For this review, take the finished solid that the model builds, in its own axes (mm). Face numbers are marked on the shaded views. A direction names the side the tool comes from. Give positions to 0.01 mm unless a question says otherwise; leave off trailing zeros. Write each loop counter-clockwise with the first axis right and the second up, starting at its lowest first coordinate (ties: lowest second). Pieces come first, ordered by that corner, then holes.
from build123d import *

# Parameters (mm, degrees)
SKETCH1_R           = 14
SKETCH1_R_2         = 7.5
BOSS_EXTRUDE1_DEPTH = 5
SKETCH2_R           = 13
SKETCH2_R_2         = 9
CUT_EXTRUDE1_DEPTH  = 0.05
FILLET1_R           = 0.45


with BuildPart() as part:
    # Sketch1 → Boss-Extrude1 (new, symmetric)
    with BuildSketch(Plane(origin=(0, 0, 0), x_dir=(1, 0, 0), z_dir=(0, 1, 0))):
        with Locations(Location((0, 0, 0), (0, 0, 270))):
            Circle(SKETCH1_R)
        with Locations(Location((0, 0, 0), (0, 0, 270))):
            Circle(SKETCH1_R_2, mode=Mode.SUBTRACT)
    extrude(amount=BOSS_EXTRUDE1_DEPTH, both=True)

    # Sketch2 → Cut-Extrude1 (cut)
    with BuildSketch(Plane(origin=(0, 5, 0), x_dir=(1, 0, 0), z_dir=(0, 1, 0))):
        with Locations(Location((0, 0, 0), (0, 0, 270))):
            Circle(SKETCH2_R)
        with Locations(Location((0, 0, 0), (0, 0, 270))):
            Circle(SKETCH2_R_2, mode=Mode.SUBTRACT)
    cut_extrude1 = extrude(amount=-CUT_EXTRUDE1_DEPTH, mode=Mode.SUBTRACT)

    # Mirror1: Cut-Extrude1 across plane
    add(cut_extrude1.mirror(Plane.ZX), mode=Mode.SUBTRACT)

    # Fillet1
    fillet1_edges = [part.edges().sort_by_distance(p)[0] for p in [
        (0, -5, -14),
        (0, 5, -14),
        (0, -5, -7.5),
        (0, 5, -7.5),
    ]]
    fillet(fillet1_edges, radius=FILLET1_R)


solid = part.part
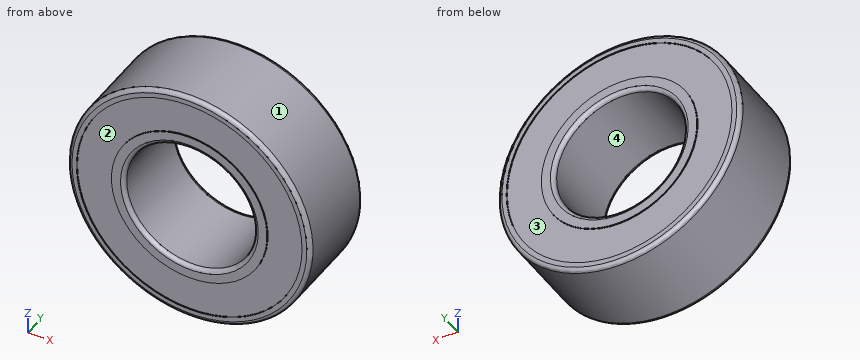
(1) Clearance check with flat-ended pins moving along their axes: pin 1 Ø15.5 at (x, z) = (0, 0) entering from +Y; pin 2 Ø3 at (x, y) = (-8, -3.5) entering from -Z; pin 3 Ø1 at (x, y) = (4, -3.5) entering from +Z. State where each tip first meets the part, or that it passes through.
(2) Tool access review of the marked faces 3 and 4: name each direction out of +Z, -Z, +X, -X, +Y, -Y from which nothing blocks a thin tool from reaching the whole face with its end or side.
(3) We need section C-C (y = -2). Write out the cut boundary in (x, z), and give its area (3 significant figures).
(4) For L1, parallel to Z at x = -0.25, y = 1.25; L2, parallel to Y at x = -7.5, z = 7, list the stretches that pass through material, from the lowest coordinate up.
(5) The part is to be moulded in two halves that separate along Z. For the marked faces 1 and 2, say which applies: +Z half, -Z half, draft (parallel to the pull), parting line (faces both ways), or undercut.
The answers:
1. pin 1: stops at y = 4.95
1. pin 2: stops at z = -12.4
1. pin 3: stops at z = 13.56
2. face 3: +Y
2. face 4: +Y, -Y
3. outline: circle Ø28 at (0, 0); hole circle Ø15 at (0, 0)
3. area: 439 mm2
4. L1: z = -14 to -7.5, 7.5 to 14
4. L2: y = -4.95 to 4.95
5. face 1: parting line
5. face 2: undercut
